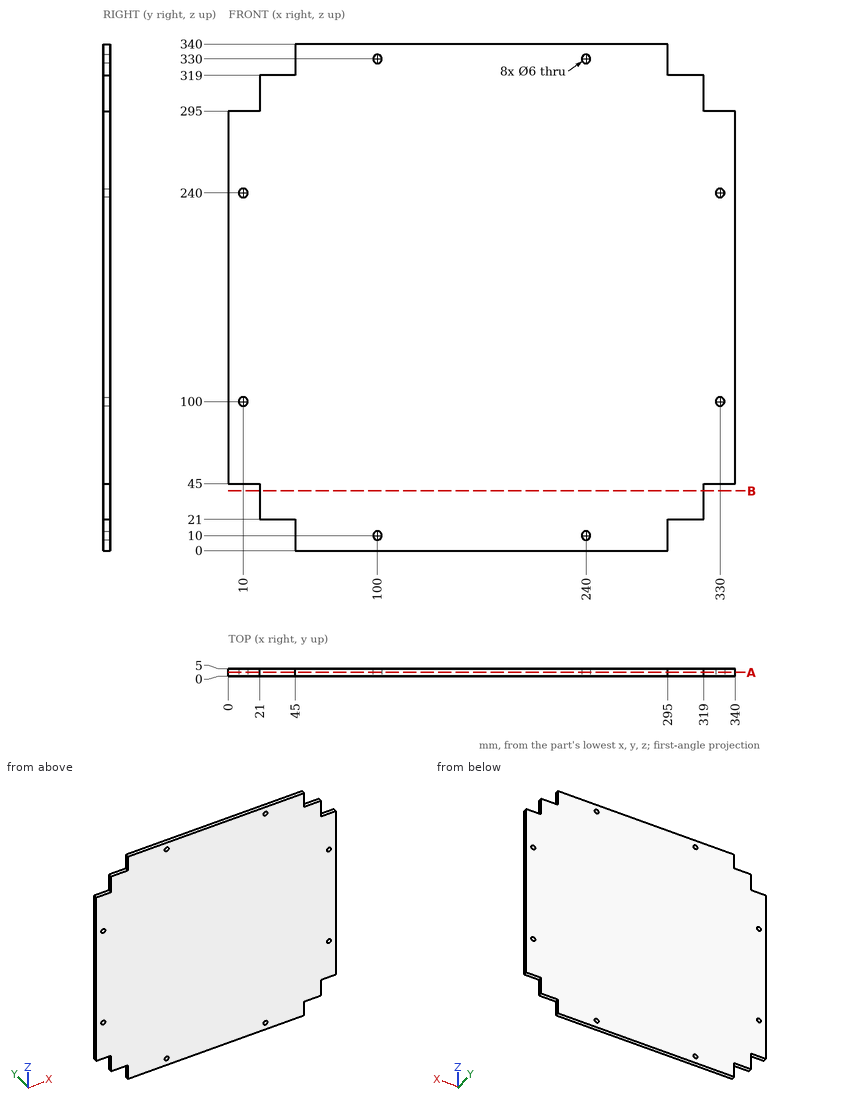
Source: three-view drawing plus pictorial views. Frame: mm from the lowest corner of the part. Coordinates: 2 decimals unless noted, no trailing zeros. Loops run counter-clockwise (first coordinate to the right, second up) from the corner with the lowest first, then second, coordinate; pieces in that order, holes last. Notation, with made-up numbers: (40.5, 85) -> (76.5, 85) arc R23 cw to (76.5, 119) -> close; hole circle Ø3 at (33, -8). An arc over 180 degrees is marked (long way). One line per item, written item: value.
(1) Cut plane A-A (y = 2.4). Give the number of separate pieces and of enclosed holes in the cut face, then the cut area to 3 significant figures.
Answer below:
separate pieces: 1
enclosed holes: 8
area: 110,000 mm2
(2) Ray query, line 1 along Z through (x, y) = (330, 3.15); line 2 along X through (y, z) = (3.55, 240). Return the intervals inside material, ascending.
Answer below:
line 1: z = 45 to 97, 103 to 237, 243 to 295
line 2: x = 0 to 7, 13 to 327, 333 to 340
(3) Pin query (flat end, axial travel): pin 1 Ø1.5 at (y, z) = (2, 32.5) entering from +X; pin 2 Ø2.5 at (x, y) = (333, 3) entering from -Z. Return the tip coordinate at first contact, or that it passes through.
Answer below:
pin 1: stops at x = 319
pin 2: stops at z = 45
(4) Cut plane B-B (z = 40). Output: boundary loops of the cut face in (x, y), then the cut area to 3 significant figures.
Answer below:
outline: (21, 0) -> (319, 0) -> (319, 5) -> (21, 5) -> close
area: 1,490 mm2
